Here's the drawing with two shaded views (mm, measured from the low corner). I have some questions. Round coordinates to 2 decimals unless told otherwise and drop trailing zeros. Loops run counter-clockwise (first coordinate to the right, second up) from the corner with the lowest first, then second, coordinate; pieces in that order, holes last.
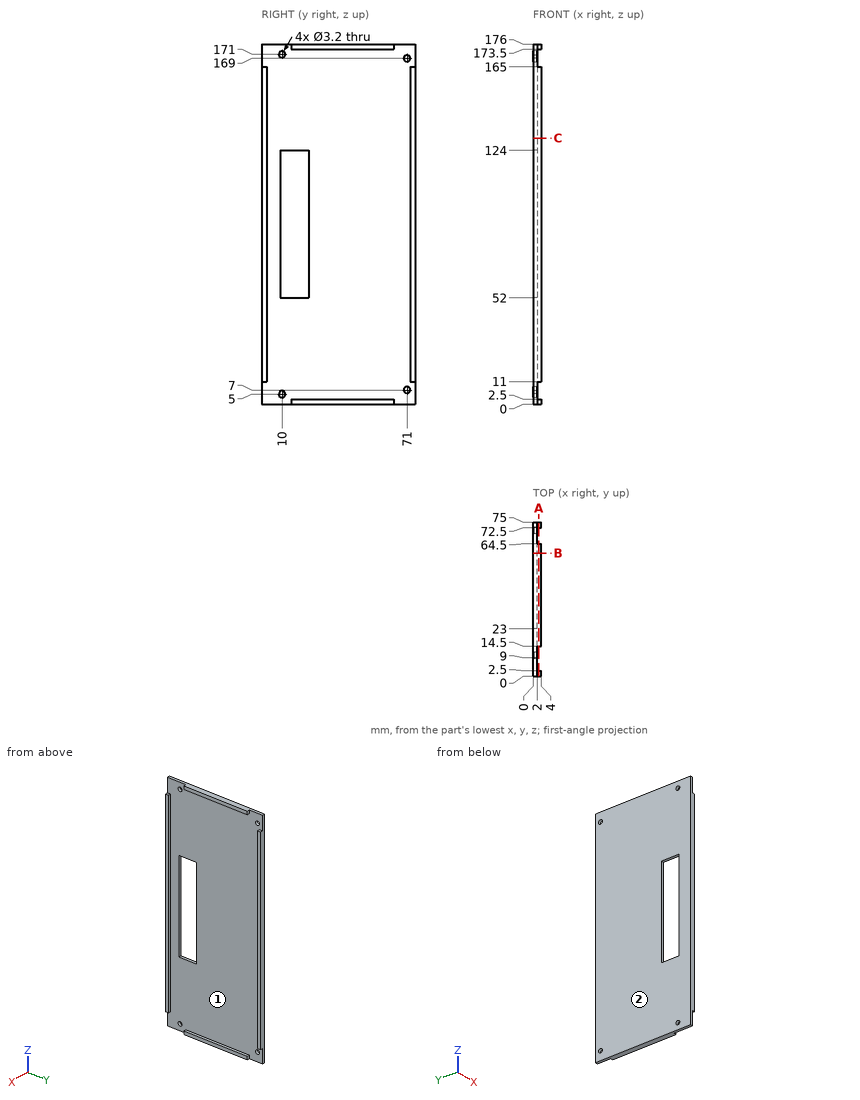
Item 1: We'd pull the mould along Y, two halves only. Please class the marked faces 1 and 2: released by +Y, released by -Y, zero draft, split by the parting line, or undercut.
Results list:
face 1: undercut
face 2: zero draft
Item 2: Will these pins go through, and if not, where does the flat tip stop? pin 1 (5 mm diameter, centred on y = 10, z = 171, fed in from +X); pin 2 (0.6 mm diameter, centred on x = 3.5, z = 175, fed in from -Y); pin 3 (2 mm diameter, centred on x = 3.5, y = 73.5, fed in from -Z).
Results list:
pin 1: stops at x = 2
pin 2: stops at y = 14.5
pin 3: stops at z = 11
Item 3: If we section it at C-C, the plane z = 130: Please give me the cut outline in (x, y).
Results list:
outline: (0, 0) - (4, 0) - (4, 2.5) - (2, 2.5) - (2, 72.5) - (4, 72.5) - (4, 75) - (0, 75) - close
Item 4: If we section it at A-A, the plane x = 2.8: Please give me the cut outline in (y, z), then the cut area to 3 significant figures.
Results list:
outline: (0, 11) - (2.5, 11) - (2.5, 165) - (0, 165) - close; (14.5, 0) - (64.5, 0) - (64.5, 2.5) - (14.5, 2.5) - close; (14.5, 173.5) - (64.5, 173.5) - (64.5, 176) - (14.5, 176) - close; (72.5, 11) - (75, 11) - (75, 165) - (72.5, 165) - close
area: 1,020 mm2
Item 5: If I drill on line 1 along Z through (x, y) = (1, 71); line 2 along Y through (x, z) = (1.65, 169); line 3 along Y through (x, z) = (0.95, 5), over which ranges is the centre line in solid material (lowest first)?
Results list:
line 1: z = 0 to 5.4, 8.6 to 167.4, 170.6 to 176
line 2: y = 0 to 69.4, 72.6 to 75
line 3: y = 0 to 8.4, 11.6 to 75
Item 6: If we section it at B-B, the plane y = 60: Please give me the cut outline in (x, z), then the cut area to 3 significant figures.
Results list:
outline: (0, 0) - (4, 0) - (4, 2.5) - (2, 2.5) - (2, 173.5) - (4, 173.5) - (4, 176) - (0, 176) - close
area: 362 mm2
